Check sheet for the modelled part. Datum: model origin and axes. Units: mm. A direction names the side the tool comes from. Give positions to 0.01 mm unless a question says otherwise; leave off trailing zeros. Order: outer loops, then holes, each group sorted by start corner. A loop starts at its lowest first (then second) coordinate and runs counter-clockwise, first axis right, second up. Notation, with made-up numbers: (7.25, 2.5) -> (49.25, 2.5) arc R14 cw to (49.25, 11.5) -> close; hole circle Ø4 at (19.5, 75.25). An arc over 180 degrees is marked (long way). Answer in a Markdown table with one row per item. Add a question column.
(1) Cross-section at B-B (x = 0). Record the cut outline in (y, z) (3 decimals).
(2) Go/stop test with flat-tipped pins: pin 1 (3.5 mm diameter, centred on x = 0, z = 0, fed in from -Y) (3 decimals); pin 2 (3 mm diameter, centred on y = 17, z = -2.5, fed in from -X). Record where each tip stops, or that it passes through.
(3) Thickness scan on L1, parallel to X at y = 3.3, z = 0; L2, parallel to X at y = 11.75, z = -1.75; L3, parallel to Y at x = 2.5, z = 0.5. Record the ranges inside material, lowest first. Write a range as [from, to].
(4) Cross-section at A-A (z = 0). Record the cut outline in (x, y) (3 decimals).
(5) Release check for a two-part mould opening along Z. For faces 1 (the face through (-3, 0, -2)), 2 (the face through (-3.905, 9.86, -0.867)), 3 (the face through (0.383, 18.486, -1.216)) record: released by +Z, released by -Z, zero draft, split by the parting line, or undercut.
(6) Set-up check for faces 4 (the face through (0.811, 10.84, -2.575)), 5 (the face through (0.736, 2.965, -2.337)), 6 (the face through (-1, 20, 2)): record each of +Z, -Z, +X, -X, +Y, -Y from which the full face is reachable in a straight line by a thin tool's end or side.
(7) Cross-section at D-D (y = 18.5). Record the cut outline in (x, z) (3 decimals).
(8) Cross-section at C-C (y = 10.25). Record the cut outline in (x, z), then the cut area to 3 significant figures.
```python
from build123d import *

# Parameters (mm, degrees)
SKETCH1_R           = 4
BOSS_EXTRUDE1_DEPTH = 20
SKETCH2_R           = 2.45
CUT_EXTRUDE1_DEPTH  = 6
SKETCH3_R           = 2.7
CUT_EXTRUDE2_DEPTH  = 10
SKETCH4_R           = 1.275
CUT_EXTRUDE3_DEPTH  = 6
CHAMFER1_SIZE       = 0.5
CHAMFER2_SIZE       = 1.5


with BuildPart() as part:
    # Sketch1 → Boss-Extrude1 (new body)
    with BuildSketch(Plane(origin=(0, 0, 0), x_dir=(1, 0, 0), z_dir=(0, 1, 0))):
        with Locations(Location((0, 0, 0), (0, 0, 270))):
            Circle(SKETCH1_R)
    extrude(amount=BOSS_EXTRUDE1_DEPTH)

    # Sketch2 → Cut-Extrude1 (cut)
    with BuildSketch(Plane.XZ):
        with Locations(Location((0, 0, 0), (0, 0, 270))):
            Circle(SKETCH2_R)
    extrude(amount=-CUT_EXTRUDE1_DEPTH, mode=Mode.SUBTRACT)

    # Sketch3 → Cut-Extrude2 (cut)
    with BuildSketch(Plane.XZ.offset(-6)):
        with Locations(Location((0, 0, 0), (0, 0, 270))):
            Circle(SKETCH3_R)
    extrude(amount=-CUT_EXTRUDE2_DEPTH, mode=Mode.SUBTRACT)

    # Sketch4 → Cut-Extrude3 (cut)
    with BuildSketch(Plane.XZ.offset(-16)):
        with Locations(Location((0, 0, 0), (0, 0, 270))):
            Circle(SKETCH4_R)
    extrude(amount=-CUT_EXTRUDE3_DEPTH, mode=Mode.SUBTRACT)

    # Chamfer1
    # the kernel refuses this chamfer: 0.5 mm, written as the material it takes off along each edge
    with BuildSketch(Plane(origin=(0, 0, 0), x_dir=(0, 0, -1), z_dir=(-1, 0, 0))) as chamfer1_piece_1:
        Polygon((2.45 + CHAMFER1_SIZE, 0), (2.45, -CHAMFER1_SIZE), (2.45, 0), align=None)
    revolve(axis=Axis((0, 0, 0), (0, -1, 0)), mode=Mode.SUBTRACT)
    with BuildSketch(Plane(origin=(0, 6, 0), x_dir=(0, 0, -1), z_dir=(-1, 0, 0))) as chamfer1_piece_2_section:
        Polygon((2.45, CHAMFER1_SIZE), (2.45 + CHAMFER1_SIZE, 0), (2.45, 0), align=None)
    chamfer1_piece_2 = revolve(axis=Axis((0, 6, 0), (0, -1, 0)), mode=Mode.PRIVATE)
    chamfer1_piece_2 = chamfer1_piece_2 & Plane(origin=(0, 5.626269224, 0), x_dir=(0, 0, -1), z_dir=(0, -1, 0)) * Cylinder(2.7, 12, mode=Mode.PRIVATE)
    add(chamfer1_piece_2, mode=Mode.SUBTRACT)
    with BuildSketch(Plane(origin=(0, 20, 0), x_dir=(0, 0, -1), z_dir=(-1, 0, 0))) as chamfer1_piece_3:
        Polygon((1.275 + CHAMFER1_SIZE, 0), (1.275, CHAMFER1_SIZE), (1.275, 0), align=None)
    revolve(axis=Axis((0, 20, 0), (0, -1, 0)), mode=Mode.SUBTRACT)

    # Chamfer2
    # the kernel refuses this chamfer: 1.5 mm, written as the material it takes off along each edge
    with BuildSketch(Plane(origin=(0, 16, 0), x_dir=(0, 0, -1), z_dir=(-1, 0, 0))) as chamfer2_piece_1_section:
        Polygon((1.275, -CHAMFER2_SIZE), (1.275 + CHAMFER2_SIZE, 0), (1.275, 0), align=None)
    chamfer2_piece_1 = revolve(axis=Axis((0, 16, 0), (0, -1, 0)), mode=Mode.PRIVATE)
    chamfer2_piece_1 = chamfer2_piece_1 & Plane(origin=(0, 16.79183668, 0), x_dir=(0, 0, -1), z_dir=(0, -1, 0)) * Cylinder(2.7, 12, mode=Mode.PRIVATE)
    add(chamfer2_piece_1, mode=Mode.SUBTRACT)


solid = part.part
```
Answer below:
| question | item | result |
|---|---|---|
| 1 | outline | (0, -4) -> (20, -4) -> (20, -1.775) -> (19.5, -1.275) -> (17.5, -1.275) -> (16.075, -2.7) -> (5.75, -2.7) -> (5.5, -2.45) -> (0.5, -2.45) -> (0, -2.95) -> close; (0, 2.95) -> (0.5, 2.45) -> (5.5, 2.45) -> (5.75, 2.7) -> (16.075, 2.7) -> (17.5, 1.275) -> (19.5, 1.275) -> (20, 1.775) -> (20, 4) -> (0, 4) -> close |
| 2 | pin 1 | stops at y = 17.025 |
| 2 | pin 2 | stops at x = -3.87 |
| 3 | L1 | x = [-4, -2.45], [2.45, 4] |
| 3 | L2 | x = [-3.6, -2.06], [2.06, 3.6] |
| 3 | L3 | y = [0.4, 5.6], [16.23, 20] |
| 4 | outline | (-4, 0) -> (-2.95, 0) -> (-2.45, 0.5) -> (-2.45, 5.5) -> (-2.7, 5.75) -> (-2.7, 16.075) -> (-1.275, 17.5) -> (-1.275, 19.5) -> (-1.775, 20) -> (-4, 20) -> close; (1.275, 17.5) -> (2.7, 16.075) -> (2.7, 5.75) -> (2.45, 5.5) -> (2.45, 0.5) -> (2.95, 0) -> (4, 0) -> (4, 20) -> (1.775, 20) -> (1.275, 19.5) -> close |
| 5 | face 1 | zero draft |
| 5 | face 2 | split by the parting line |
| 5 | face 3 | undercut |
| 6 | face 4 | none |
| 6 | face 5 | -Y |
| 6 | face 6 | +Z, -Z, +X, -X, +Y |
| 7 | outline | circle Ø8 at (0, 0); hole circle Ø2.55 at (0, 0) |
| 8 | outline | circle Ø8 at (0, 0); hole circle Ø5.4 at (0, 0) |
| 8 | area | 27.4 mm² |
